Input: part model. Units: mm. Frame: model coordinates. A direction names the side the tool comes from. Round coordinates to 2 decimals unless told otherwise and drop trailing zeros. Loops run counter-clockwise (first coordinate to the right, second up) from the corner with the lowest first, then second, coordinate; pieces in that order, holes last. Notation, with made-up numbers: M -37.75,-39.5 L -31.75,-39.5 A16 ccw -31.75,-11.5 Z; hole C -8,54 d4. An arc over 180 degrees is marked long. Return JSON: item names as keys, results as strings. Group by question number.
1) Section B-B (z = 18.5). Output: boundary loops of the cut face in (x, y), plus the area to 3 significant figures.
2) Section C-C (y = 39). Output: boundary loops of the cut face in (x, z).
3) Section D-D (x = 40). Output: boundary loops of the cut face in (y, z).
4) Material intervals for line 1 (X direction, y = 31, z = 23); line 2 (X direction, y = 8, z = 22.5); line 3 (Y direction, x = 11.5, z = 48), sorted ascending. Write a range as from..to.
5) Contact query for flat-ended pins moving along their axis: P1, Ø1, axis at x = 43.5, z = 21, coming from the -Y side; P2, Ø10, axis at y = 18, z = 14, coming from the +X side; P3, Ø12, axis at x = 49, y = 41, coming from the +Z side; P4, Ø4, axis at y = 45.5, z = 33.5, coming from the -X side. Output: stop coordinate, or through.
6) Access query for faces 1 (the face through (47, 38.1, 19)), 2 (the face through (57.15, 44, 13)), 3 (the face through (12.7, 45, 25)), 4 (the face through (6, 12.7, 25)). Directions: +Z, -Z, +X, -X, +Y, -Y. A direction counts if a zero-diameter tool reaches every point of the face in a straight line with its end or side. Return the directions, or none.
7) Section A-A (x = 50.5). Output: boundary loops of the cut face in (y, z), plus the area to 3 significant figures.
from build123d import *

# Parameters (mm, degrees)
F1_DEPTH = 50.8
F3_DEPTH = 50.8
F4_W     = 19.05
F4_H     = 25.4
F5_DEPTH = 38.1


with BuildPart() as f1:
    # F0 (on Top) → F1 (new body)
    with BuildSketch(Plane.XY):
        Polygon((12.7, 12.7), (12.7, 0), (25.4, 0), (25.4, 50.8), (12.7, 50.8), (12.7, 38.1), (0, 38.1), (0, 12.7), align=None)
    extrude(amount=F1_DEPTH)

    # F2 (on Front) → F3 (join)
    with BuildSketch(Plane.XZ):
        Polygon((25.4, 50.8), (25.4, 0), (57.15, 0), (57.15, 25.4), (38.1, 50.8), align=None)
    extrude(amount=-F3_DEPTH)

    # F4 (on Top) → F5 (cut)
    with BuildSketch(Plane.XY):
        with Locations((47.625, 25.4)):
            Rectangle(F4_W, F4_H)
    extrude(amount=F5_DEPTH, mode=Mode.SUBTRACT)


solid = f1.part
Returned:
{
 "1": {"outline": "M 0,12.7 L 12.7,12.7 L 12.7,0 L 57.15,0 L 57.15,12.7 L 38.1,12.7 L 38.1,38.1 L 57.15,38.1 L 57.15,50.8 L 12.7,50.8 L 12.7,38.1 L 0,38.1 Z", "area": "2,100 mm^2"},
 "2": {"outline": "M 12.7,0 L 57.15,0 L 57.15,25.4 L 38.1,50.8 L 12.7,50.8 Z"},
 "3": {"outline": "M 0,0 L 12.7,0 L 12.7,38.1 L 38.1,38.1 L 38.1,0 L 50.8,0 L 50.8,48.27 L 0,48.27 Z"},
 "4": {"line 1": "x = 0..38.1", "line 2": "x = 12.7..57.15", "line 3": "y = 12.7..38.1"},
 "5": {"P1": "stops at y = 0", "P2": "stops at x = 38.1", "P3": "stops at z = 44.27", "P4": "stops at x = 12.7"},
 "6": {"face 1": "-Z, +X", "face 2": "+Z, -Z, +X, +Y, -Y", "face 3": "+Z, -Z, -X, +Y", "face 4": "+Z, -Z, -X, -Y"},
 "7": {"outline": "M 0,0 L 12.7,0 L 12.7,34.27 L 0,34.27 Z; M 38.1,0 L 50.8,0 L 50.8,34.27 L 38.1,34.27 Z", "area": "870 mm^2"}
}
